For this review, take the finished solid that the model builds, in its own axes (mm). A direction names the side the tool comes from. Round coordinates to 2 decimals unless told otherwise and drop trailing zeros. Write each loop counter-clockwise with the first axis right and the second up, starting at its lowest first coordinate (ties: lowest second). Pieces come first, ordered by that corner, then holes. Notation, with made-up numbers: (44.25, 65) - (84.25, 65) arc R16 cw to (84.25, 89) - close; hole circle Ø5 at (7.25, 87). An arc over 180 degrees is marked (long way). One line per item, written item: value. Start each with the question number.
Q1. Add section B-B on x = 18. Write out the cut boundary in (y, z), and give its area (3 significant figures).
Q2. For probe 1 along Z at (x, y) = (-114, -28); probe 2 along Z at (x, y) = (-55.5, 0.5); probe 3 along Y at (x, z) = (40.5, 230.5), list the stretches that pass through material, from the lowest coordinate up.
Q3. Mouldability with a two-part tool opening along Z and no side actions: class faces 4 (the face through (-54.73, -13.66, 200.19)), 5 (the face through (-28, 37.328, 228)), 6 (the face through (-29, -37, 0)) as +Z half, -Z half, draft (parallel to the pull), parting line (faces both ways), or undercut.
Q4. Add section D-D on x = -4.5. Write out the cut boundary in (y, z).
Q5. Add section A-A on y = -83. Write out the cut boundary in (x, z), and give its area (3 significant figures).
Q6. Add section C-C on y = 48.5. Write out the cut boundary in (x, z).
Q7. Clearance check with flat-ended pins moving along their axes: pin 1 Ø2 at (x, z) = (5, 59) entering from +Y; pin 2 Ø1.5 at (y, z) = (-74.5, 167.5) entering from -X; pin 3 Ø12 at (x, z) = (-53, 226.5) entering from -Y. State where each tip first meets the part, or that it passes through.
Q8. Tool access review of faces 1 (the face through (19, -37, 201.2)), 2 (the face through (46.623, -40, 228)), 3 (the face through (-28, -115.332, 228)): name each direction out of +Z, -Z, +X, -X, +Y, -Y from which nothing blocks a thin tool from reaching the whole face with its end or side.
```python
from build123d import *

# Parameters (mm, degrees)
F0_R     = 107.95
F1_DEPTH = 199.2
F2_R     = 37.5
F3_DEPTH = 2
F4_R     = 107.95
F5_DEPTH = 2
F6_W     = 147.4276631508
F6_H     = 152.66
F7_DEPTH = 50


with BuildPart() as f1:
    # F0 (on Top) → F1 (new body)
    with BuildSketch(Plane.XY):
        with Locations((-27.0904134959, -39.0018522739)):
            Circle(F0_R)
    extrude(amount=F1_DEPTH)

    # F2 (on face) → F3 (join)
    with BuildSketch(Plane.XY.offset(199.2)):
        with Locations((-27.0904134959, -39.0018522739)):
            Circle(F2_R)
    extrude(amount=F3_DEPTH)

    # F4 (on face) → F5 (join)
    with BuildSketch(Plane.XY.offset(201.2)):
        with Locations((-27.0904134959, -39.0018522739)):
            Circle(F4_R)
    extrude(amount=F5_DEPTH)

    # F6 (on face) → F7 (join)
    with BuildSketch(Plane.XY.offset(203.2)):
        with Locations((-27.0904134959, -39.0018522739)):
            Rectangle(F6_W, F6_H)
    extrude(amount=F7_DEPTH)


solid = f1.part
```
Result set:
1. outline: (-137.08, 0) - (59.08, 0) - (59.08, 199.2) - (-137.08, 199.2) - close; (-137.08, 201.2) - (59.08, 201.2) - (59.08, 203.2) - (37.33, 203.2) - (37.33, 253.2) - (-115.33, 253.2) - (-115.33, 203.2) - (-137.08, 203.2) - close
1. area: 47,100 mm^2
2. probe 1: z = 0 to 199.2, 201.2 to 203.2
2. probe 2: z = 0 to 199.2, 201.2 to 253.2
2. probe 3: y = -115.33 to 37.33
3. face 4: undercut
3. face 5: draft
3. face 6: -Z half
4. outline: (-144.56, 0) - (66.56, 0) - (66.56, 199.2) - (-9.07, 199.2) - (-9.07, 201.2) - (66.56, 201.2) - (66.56, 203.2) - (37.33, 203.2) - (37.33, 253.2) - (-115.33, 253.2) - (-115.33, 203.2) - (-144.56, 203.2) - (-144.56, 201.2) - (-68.93, 201.2) - (-68.93, 199.2) - (-144.56, 199.2) - close
5. outline: (-125.67, 0) - (71.49, 0) - (71.49, 199.2) - (-125.67, 199.2) - close; (-125.67, 201.2) - (71.49, 201.2) - (71.49, 203.2) - (46.62, 203.2) - (46.62, 253.2) - (-100.8, 253.2) - (-100.8, 203.2) - (-125.67, 203.2) - close
5. area: 47,000 mm^2
6. outline: (-90.31, 0) - (36.13, 0) - (36.13, 199.2) - (-90.31, 199.2) - close; (-90.31, 201.2) - (36.13, 201.2) - (36.13, 203.2) - (-90.31, 203.2) - close
7. pin 1: stops at y = 64.37
7. pin 2: stops at x = -129.29
7. pin 3: stops at y = -115.33
8. face 1: none
8. face 2: +Z, +X, +Y, -Y
8. face 3: +Z, +X, -X, -Y
